from build123d import *

# Parameters (mm, degrees)
BOSS_EXTRUDE2_DEPTH = 107
BOSS_EXTRUDE3_DEPTH = 107
CUT_EXTRUDE4_DEPTH  = 104.5
SKETCH4_W           = 4
SKETCH4_H           = 2
BOSS_EXTRUDE4_DEPTH = 104.5
SKETCH6_W           = 42
SKETCH6_H           = 13
CUT_EXTRUDE5_DEPTH  = 3
SKETCH7_W           = 12
SKETCH7_H           = 7
CUT_EXTRUDE6_DEPTH  = 3
SKETCH8_W           = 72
SKETCH8_H           = 26
CUT_EXTRUDE7_DEPTH  = 3
SKETCH9_R           = 1.85
CUT_EXTRUDE8_DEPTH  = 3


with BuildPart() as part:
    # Sketch1 → Boss-Extrude2 (new body)
    with BuildSketch(Plane(origin=(0, 0, 0), x_dir=(0, 0, -1), z_dir=(1, 0, 0))):
        Polygon((-70, 49.18258427), (-32, 49.18258427), (0, 12.18258427), (0, -4.81741573), (-70, -4.81741573), align=None)
    extrude(amount=BOSS_EXTRUDE2_DEPTH)

    # Sketch2 → Boss-Extrude3 (add)
    with BuildSketch(Plane(origin=(107, 0, 0), x_dir=(0, 0, -1), z_dir=(1, 0, 0))):
        Polygon((-72.5, -7.31741573), (-72.5, 51.68258427), (-30.856871673, 51.68258427), (2.5, 13.113701397), (2.5, -7.31741573), align=None)
        Polygon((-70, 49.18258427), (-32, 49.18258427), (0, 12.18258427), (0, -4.81741573), (-70, -4.81741573), align=None, mode=Mode.SUBTRACT)
    extrude(amount=-BOSS_EXTRUDE3_DEPTH)

    # Sketch3 → Cut-Extrude4 (cut)
    with BuildSketch(Plane(origin=(107, 0, 0), x_dir=(0, 0, -1), z_dir=(1, 0, 0))):
        Polygon((0, -4.81741573), (-70, -4.81741573), (-70, 49.18258427), (-32, 49.18258427), (0, 12.18258427), align=None)
    extrude(amount=-CUT_EXTRUDE4_DEPTH, mode=Mode.SUBTRACT)

    # Sketch4 → Boss-Extrude4 (add)
    with BuildSketch(Plane(origin=(2.5, 0, 0), x_dir=(0, 0, -1), z_dir=(1, 0, 0))):
        with Locations((-68, -3.81741573)):
            Rectangle(SKETCH4_W, SKETCH4_H)
        with Locations((-2, -3.81741573)):
            Rectangle(SKETCH4_W, SKETCH4_H)
    extrude(amount=BOSS_EXTRUDE4_DEPTH)

    # Sketch6 → Cut-Extrude5 (cut)
    with BuildSketch(Plane.XY.offset(72.5)):
        with Locations((31.5, 3.78258427)):
            Rectangle(SKETCH6_W, SKETCH6_H)
    extrude(amount=-CUT_EXTRUDE5_DEPTH, mode=Mode.SUBTRACT)

    # Sketch7 → Cut-Extrude6 (cut)
    with BuildSketch(Plane.XY.offset(72.5)):
        with Locations((79.5, 0.68258427)):
            Rectangle(SKETCH7_W, SKETCH7_H)
    extrude(amount=-CUT_EXTRUDE6_DEPTH, mode=Mode.SUBTRACT)

    # Sketch8 → Cut-Extrude7 (cut)
    with BuildSketch(Plane(origin=(0, 6.848487351, -7.9185635), x_dir=(-1, 0, 0), z_dir=(0, 0.654151933, -0.756363172))):
        with Locations((-53.5, 34.775885648)):
            Rectangle(SKETCH8_W, SKETCH8_H)
    extrude(amount=-CUT_EXTRUDE7_DEPTH, mode=Mode.SUBTRACT)

    # Sketch9 → Cut-Extrude8 (cut)
    with BuildSketch(Plane(origin=(0, 6.848487351, -7.9185635), x_dir=(-1, 0, 0), z_dir=(0, 0.654151933, -0.756363172))):
        with Locations((-91.606829089, 51.125885648)):
            Circle(SKETCH9_R)
        with Locations((-15.406829089, 51.125885648)):
            Circle(SKETCH9_R)
        with Locations((-15.406829089, 18.425885648)):
            Circle(SKETCH9_R)
        with Locations((-91.606829089, 18.425885648)):
            Circle(SKETCH9_R)
    extrude(amount=-CUT_EXTRUDE8_DEPTH, mode=Mode.SUBTRACT)


solid = part.part
Read the model definition and answer for the solid it produces. Units are mm, in the model's axes. A direction names the side the tool comes from. Give positions to 0.01 mm unless a question says otherwise; leave off trailing zeros. Loops run counter-clockwise (first coordinate to the right, second up) from the corner with the lowest first, then second, coordinate; pieces in that order, holes last. Notation, with made-up numbers: (5, 69.25) -> (42, 69.25) arc R17 ccw to (42, 98.25) -> close; hole circle Ø8 at (26, 13.25). An arc over 180 degrees is marked (long way). Use a Markdown table: item, result.
Q1. Section B-B, the plane x = 40.5 is taken. Determine the outline of the cut face in (y, z), then the cut area to 3 significant figures.
Solved:
| item | result |
|---|---|
| outline | (-7.32, -2.5) -> (13.11, -2.5) -> (23.32, 6.33) -> (21.68, 8.22) -> (12.18, 0) -> (-2.82, 0) -> (-2.82, 4) -> (-4.82, 4) -> (-4.82, 66) -> (-2.82, 66) -> (-2.82, 70) -> (-2.72, 70) -> (-2.72, 72.5) -> (-7.32, 72.5) -> close; (10.28, 70) -> (49.18, 70) -> (49.18, 32) -> (41.35, 25.23) -> (42.98, 23.33) -> (51.68, 30.86) -> (51.68, 72.5) -> (10.28, 72.5) -> close |
| area | 512 mm^2 |
Q2. Determine the mould class of faces 4 (the face through (54.25, 19.81, 3.29)), 5 (the face through (13.642, 20.399, 5.43)), 6 (the face through (107, -6, 41)) for opening direction Y: pulls with the +Y half, pulls with the -Y half, needs draft (parallel to the pull), parting line crosses it, or undercut.
Solved:
| item | result |
|---|---|
| face 4 | pulls with the +Y half |
| face 5 | undercut |
| face 6 | needs draft |
Q3. Find the intervals of material crossed by line 1 along Z through (x, y) = (93.5, -4.5); line 2 along Y through (x, z) = (88, 41); line 3 along Z through (x, y) = (61, 7), in increasing order.
Solved:
| item | result |
|---|---|
| line 1 | z = -2.5 to 4, 66 to 72.5 |
| line 2 | y = -7.32 to -4.82, 49.18 to 51.68 |
| line 3 | z = -2.5 to 0, 70 to 72.5 |
Q4. Section D-D, the plane x = 70 is taken. Determine the outline of the cut face in (y, z), then the cut area to 3 significant figures.
Solved:
| item | result |
|---|---|
| outline | (-7.32, -2.5) -> (13.11, -2.5) -> (23.32, 6.33) -> (21.68, 8.22) -> (12.18, 0) -> (-2.82, 0) -> (-2.82, 4) -> (-4.82, 4) -> (-4.82, 66) -> (-2.82, 66) -> (-2.82, 70) -> (49.18, 70) -> (49.18, 32) -> (41.35, 25.23) -> (42.98, 23.33) -> (51.68, 30.86) -> (51.68, 72.5) -> (-7.32, 72.5) -> close |
| area | 545 mm^2 |
Q5. Section A-A, the plane y = 5.5 is taken. Determine the outline of the cut face in (x, z).
Solved:
| item | result |
|---|---|
| outline | (0, -2.5) -> (107, -2.5) -> (107, 0) -> (2.5, 0) -> (2.5, 70) -> (10.5, 70) -> (10.5, 72.5) -> (0, 72.5) -> close; (52.5, 70) -> (107, 70) -> (107, 72.5) -> (52.5, 72.5) -> close |
Q6. Section C-C, the plane z = 57 is taken. Determine the outline of the cut face in (x, y), then the cut area to 3 significant figures.
Solved:
| item | result |
|---|---|
| outline | (0, -7.32) -> (107, -7.32) -> (107, -4.82) -> (2.5, -4.82) -> (2.5, 49.18) -> (107, 49.18) -> (107, 51.68) -> (0, 51.68) -> close |
| area | 670 mm^2 |
Q7. A tool of negligible diameter and unlimited length cuts with its end or side. For faces 1 (the face through (13.698, 44.176, 25.994)), 2 (the face through (85.5, 1, 71)), 3 (the face through (54, -2.817, 2)), from which of +Z, -Z, +X, -X, +Y, -Y can it reach the whole face along a straight path? Write none if from no direction.
Solved:
| item | result |
|---|---|
| face 1 | none |
| face 2 | +Z |
| face 3 | +X |
Q8. Each of these flat-tipped pins is pushed along its axis until it touches: pin 1 (4.5 mm diameter, centred on x = 72.5, z = 2, fed in from +Y); pin 2 (2 mm diameter, centred on y = 24, z = 57, fed in from +X); pin 3 (1.5 mm diameter, centred on x = 55.5, y = 30.5, fed in from -Z). Where does it stop, or does it pass through?
Solved:
| item | result |
|---|---|
| pin 1 | stops at y = 20.92 |
| pin 2 | stops at x = 2.5 |
| pin 3 | stops at z = 70 |
